Check sheet for the drawn part. Datum: minimum x, y, z corner. Units: mm. A direction names the side the tool comes from. Give positions to 0.01 mm unless a question says otherwise; leave off trailing zeros. Write each loop counter-clockwise with the first axis right and the second up, starting at its lowest first coordinate (ties: lowest second). Pieces come first, ordered by that corner, then holes. Notation, with made-up numbers: (11, 17) - (25, 17) arc R18 ccw to (25, 46) - close; hole circle Ø11 at (31, 30). An arc over 180 degrees is marked (long way). Use a Markdown table: item, result.
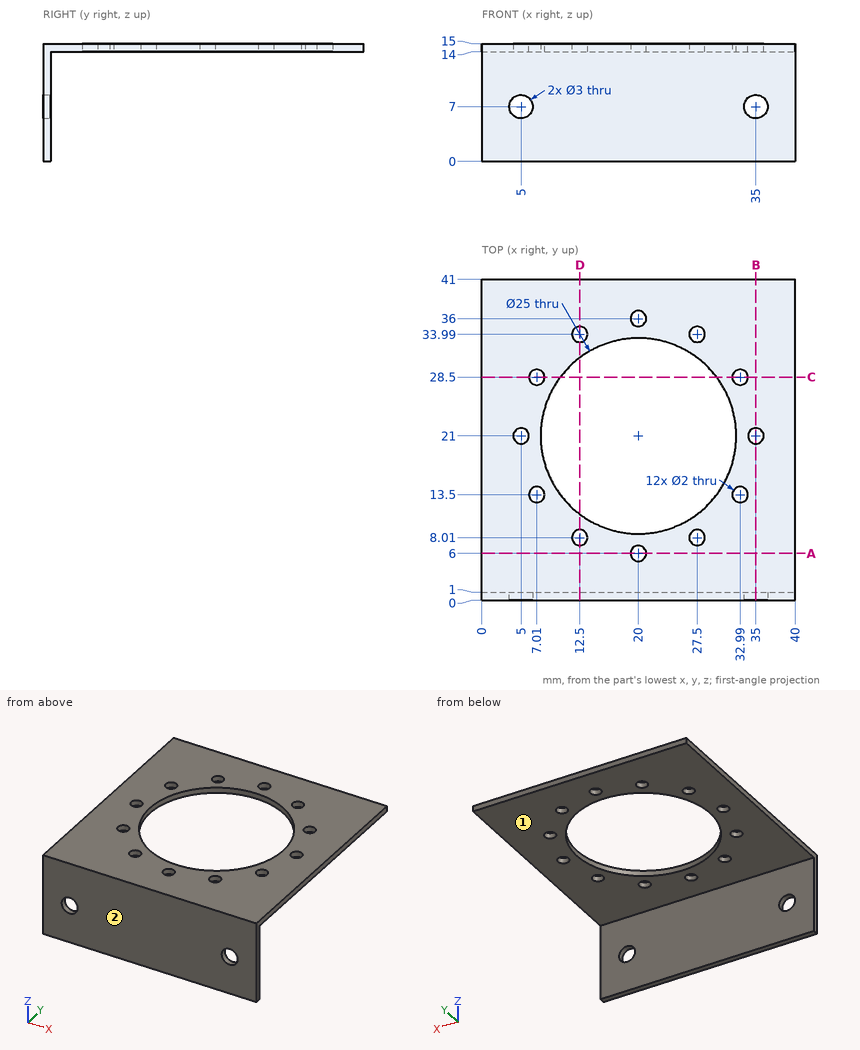
1) Set-up check for the marked faces 1 and 2: record each of +Z, -Z, +X, -X, +Y, -Y from which the full face is reachable in a straight line by a thin tool's end or side.
Working result:
| item | result |
|---|---|
| face 1 | -Z, +X, -X, +Y |
| face 2 | +Z, -Z, +X, -X, -Y |
2) Section check C-C on y = 28.5. Record the boundary of the cut face in (x, z), then the cut area to 3 significant figures.
Working result:
| item | result |
|---|---|
| outline | (0, 14) - (6.01, 14) - (6.01, 15) - (0, 15) - close; (8.01, 14) - (10, 14) - (10, 15) - (8.01, 15) - close; (30, 14) - (31.99, 14) - (31.99, 15) - (30, 15) - close; (33.99, 14) - (40, 14) - (40, 15) - (33.99, 15) - close |
| area | 16.0 mm² |
3) Section check A-A on y = 6. Record the boundary of the cut face in (x, z).
Working result:
| item | result |
|---|---|
| outline | (0, 14) - (19, 14) - (19, 15) - (0, 15) - close; (21, 14) - (40, 14) - (40, 15) - (21, 15) - close |
4) Section check D-D on x = 12.5. Record the boundary of the cut face in (y, z).
Working result:
| item | result |
|---|---|
| outline | (0, 0) - (1, 0) - (1, 14) - (7.01, 14) - (7.01, 15) - (0, 15) - close; (9.01, 14) - (11, 14) - (11, 15) - (9.01, 15) - close; (31, 14) - (32.99, 14) - (32.99, 15) - (31, 15) - close; (34.99, 14) - (41, 14) - (41, 15) - (34.99, 15) - close |
5) Section check B-B on x = 35. Record the boundary of the cut face in (y, z).
Working result:
| item | result |
|---|---|
| outline | (0, 0) - (1, 0) - (1, 5.5) - (0, 5.5) - close; (0, 8.5) - (1, 8.5) - (1, 14) - (20, 14) - (20, 15) - (0, 15) - close; (22, 14) - (41, 14) - (41, 15) - (22, 15) - close |
6) Material ranges on L1, parallel to Y at x = 20, z = 14.45; L2, parallel to X at y = 0.65, z = 7; L3, parallel to X at y = 36, z = 14.6, recorded low to high. Write a range as from..to.
Working result:
| item | result |
|---|---|
| L1 | y = 0..5, 7..8.5, 33.5..35, 37..41 |
| L2 | x = 0..3.5, 6.5..33.5, 36.5..40 |
| L3 | x = 0..19, 21..40 |
7) Depth check by flat-ended pin: P1, Ø1.6, axis at x = 7.01, y = 13.5, coming from the +Z side (3 decimals); P2, Ø2.5, axis at x = 35, y = 21, coming from the -Z side; P3, Ø1.5, axis at x = 5.5, z = 3.5, coming from the +Y side. Enter the tip coordinate at first touch or a pass-through.
Working result:
| item | result |
|---|---|
| P1 | passes through |
| P2 | stops at z = 14 |
| P3 | stops at y = 1 |
